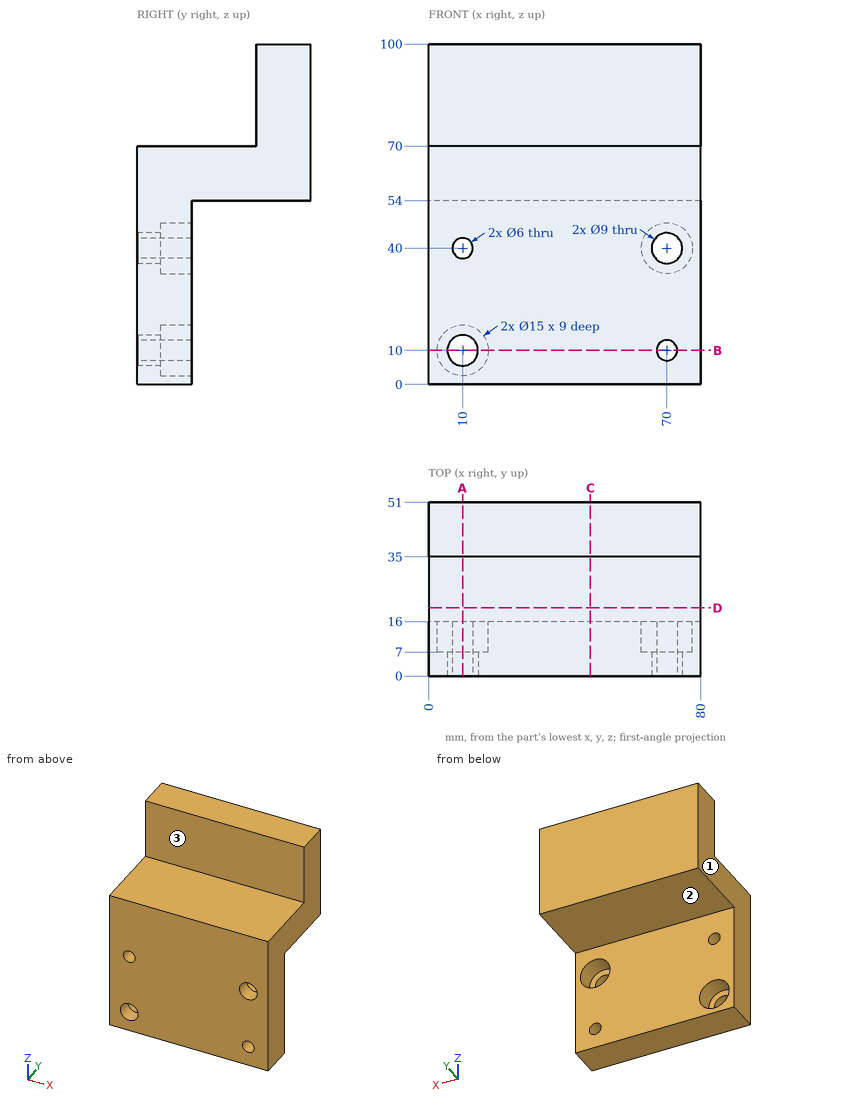
The drawing under review shows one solid part. Ordinate dimensions are in mm from its lowest x, y, z. A direction names the side the tool comes from. Coordinates: 2 decimals unless noted, no trailing zeros. Loops run counter-clockwise (first coordinate to the right, second up) from the corner with the lowest first, then second, coordinate; pieces in that order, holes last. Notation, with made-up numbers: (45.5, 49) - (62.5, 49) arc R18 cw to (62.5, 60) - close; hole circle Ø11 at (-28, 79). An arc over 180 degrees is marked (long way). Use CSV: the item, a comma, the result in double quotes. Start each with the question number.
1. To check wall thickness, follow probe 1 along X at (y, z) = (3.5, 40); probe 2 along X at (y, z) = (9.5, 40); probe 3 along Z at (x, y) = (70, 11). State the ranges of each line that lie inside material, in increasing order.
2. Clearance check with flat-ended pins moving along their axes: pin 1 (16 mm diameter, centred on x = 40, z = 20.5, fed in from +Y); pin 2 (3 mm diameter, centred on y = 17.5, z = 64, fed in from -X); pin 3 (9 mm diameter, centred on x = 48.5, z = 85.5, fed in from -Y); pin 4 (14.5 mm diameter, centred on x = 70, z = 40, fed in from +Y). State where each tip first meets the part, or that it passes through.
3. Add section D-D on y = 20. Give the boundary of the cut face in (x, z), plus the area to 3 significant figures.
4. Add section C-C on x = 47.5. Give the boundary of the cut face in (y, z).
5. For the marked faces 1, 2 and 3, list the 3-axis set-ups (+Z, -Z, +X, -X, +Y, -Y) from which the entire face can be reached by the end or side of a thin tool; tool diameter is ignored.
6. Add section B-B on z = 10. Give the boundary of the cut face in (x, y).
7. Add section A-A on x = 10. Give the boundary of the cut face in (y, z).
Resolved:
1,probe 1,"0 to 7, 13 to 65.5, 74.5 to 80"
1,probe 2,"0 to 7, 13 to 62.5, 77.5 to 80"
1,probe 3,"0 to 7, 13 to 32.5, 47.5 to 70"
2,pin 1,"y = 16"
2,pin 2,"x = 0"
2,pin 3,"y = 35"
2,pin 4,"y = 7"
3,outline,"(0, 54) - (80, 54) - (80, 70) - (0, 70) - close"
3,area,"1,280 mm2"
4,outline,"(0, 0) - (16, 0) - (16, 54) - (51, 54) - (51, 100) - (35, 100) - (35, 70) - (0, 70) - close"
5,face 1,"+Z, -Z, -X, +Y, -Y"
5,face 2,"-Z, +X, -X, +Y"
5,face 3,"+Z, +X, -X, -Y"
6,outline,"(0, 0) - (5.5, 0) - (5.5, 7) - (2.5, 7) - (2.5, 16) - (0, 16) - close; (14.5, 0) - (67, 0) - (67, 16) - (17.5, 16) - (17.5, 7) - (14.5, 7) - close; (73, 0) - (80, 0) - (80, 16) - (73, 16) - close"
7,outline,"(0, 0) - (16, 0) - (16, 2.5) - (7, 2.5) - (7, 5.5) - (0, 5.5) - close; (0, 14.5) - (7, 14.5) - (7, 17.5) - (16, 17.5) - (16, 37) - (0, 37) - close; (0, 43) - (16, 43) - (16, 54) - (51, 54) - (51, 100) - (35, 100) - (35, 70) - (0, 70) - close"
